from build123d import *

# Parameters (mm, degrees)
F0_R     = 2
F1_DEPTH = 1
F2_R     = 1.35
F3_DEPTH = 24.892
F4_R     = 1.560852
F4_R_2   = 1.35
F5_DEPTH = 0.1016
F7_DEPTH = 11.43


with BuildPart() as f1:
    # F0 (on Top) → F1 (new body)
    with BuildSketch(Plane.XY):
        with Locations((-9.958773, 15.992578)):
            Circle(F0_R)
    extrude(amount=F1_DEPTH)

    # F2 (on face) → F3 (join)
    with BuildSketch(Plane.XY):
        with Locations((-9.925794, 16.001273)):
            Circle(F2_R)
    extrude(amount=F3_DEPTH)

    # F4 (on face) → F5 (join)
    with BuildSketch(Plane.XY.offset(24.892)):
        with Locations((-9.925794, 16.001273)):
            Circle(F4_R)
        with Locations((-9.925794, 16.001273)):
            Circle(F4_R_2, mode=Mode.SUBTRACT)
    extrude(amount=-F5_DEPTH)

    # F6 (on face) → F7 (cut)
    with BuildSketch(Plane.XY.offset(24.892)):
        with BuildLine():
            ThreePointArc((-10.292375, 14.484079), (-9.925794, 14.440421), (-9.559213, 14.484079))
            Line((-9.559213, 14.484079), (-9.559213, 17.518467))
            ThreePointArc((-9.559213, 17.518467), (-9.925794, 17.562125), (-10.292375, 17.518467))
            Line((-10.292375, 17.518467), (-10.292375, 14.484079))
        make_face()
    extrude(amount=-F7_DEPTH, mode=Mode.SUBTRACT)


solid = f1.part
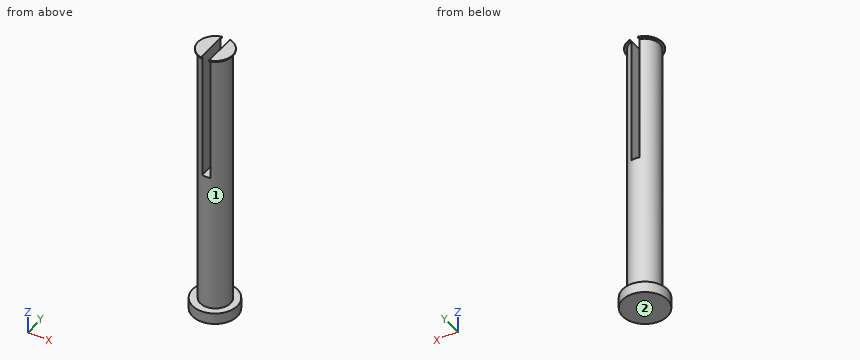
Design review of the part built by this model. Coordinates are the model's own, in mm. Face numbers are marked on the shaded views. Give positions to 0.01 mm unless a question says otherwise; leave off trailing zeros. Order: outer loops, then holes, each group sorted by start corner. A loop starts at its lowest first (then second) coordinate and runs counter-clockwise, first axis right, second up.
1. Mouldability with a two-part tool opening along Z and no side actions: class the marked faces 1 and 2 as +Z half, -Z half, draft (parallel to the pull), parting line (faces both ways), or undercut.
Solution:
face 1: undercut
face 2: -Z half
2. Add section D-D, the plane x = -10.05. State the section outline as (y, z) points.
Solution:
outline: (13.99, 0) - (17.99, 0) - (17.99, 1) - (17.35, 1) - (17.35, 13.46) - (14.66, 13.46) - (14.66, 1) - (13.99, 1) - close
3. To check wall thickness, follow L1, parallel to X at y = 15.9, z = 21; L2, parallel to Y at x = -9.85, z = 11.25; L3, parallel to Z at x = -9.65, y = 15. State the ranges of each line that lie inside material, in increasing order.
Solution:
L1: x = -11.27 to -10.29, -9.56 to -8.58
L2: y = 14.65 to 17.35
L3: z = 0 to 13.46
4. Add section A-A, the plane x = -9.15. State the section outline as (y, z) points.
Solution:
outline: (14.16, 0) - (17.82, 0) - (17.82, 1) - (17.11, 1) - (17.11, 24.79) - (17.36, 24.79) - (17.36, 24.89) - (14.65, 24.89) - (14.65, 24.79) - (14.9, 24.79) - (14.9, 1) - (14.16, 1) - close
5. For pin 1 Ø1 at (y, z) = (16.5, 17.5) entering from -X; pin 2 Ø2 at (x, z) = (-9, 21.5) entering from +Y; pin 3 Ø1 at (y, z) = (14.5, 4.5) entering from -X, all flat-tipped, find the tip position at first contact; note any pin that passes through.
Solution:
pin 1: stops at x = -11.28
pin 2: stops at y = 17.3
pin 3: stops at x = -10.83
6. Add section B-B, the plane y = 15.3. State the section outline as (x, z) points, then the cut area to 3 significant figures.
Solution:
outline: (-11.84, 0) - (-8.08, 0) - (-8.08, 1) - (-8.77, 1) - (-8.77, 24.79) - (-8.53, 24.79) - (-8.53, 24.89) - (-9.56, 24.89) - (-9.56, 13.46) - (-10.29, 13.46) - (-10.29, 24.89) - (-11.32, 24.89) - (-11.32, 24.79) - (-11.08, 24.79) - (-11.08, 1) - (-11.84, 1) - close
area: 50.5 mm2
7. Add section C-C, the plane z = 21. State the section outline as (x, y) points.
Solution:
outline: (-10.29, 14.7) - (-10.29, 17.3) arc R1.35 ccw to start; (-9.56, 14.7) arc R1.35 ccw to (-9.56, 17.3) - close
